Design review of the part built by this model. Coordinates are the model's own, in mm. Give positions to 0.01 mm unless a question says otherwise; leave off trailing zeros. Loops run counter-clockwise (first coordinate to the right, second up) from the corner with the lowest first, then second, coordinate; pieces in that order, holes last. Notation, with made-up numbers: M 55,51 L 111,51 A24 cw 111,63 Z; hole C -17.75,3.5 d7. An arc over 180 degrees is marked long. Answer as CSV lines item,"result".
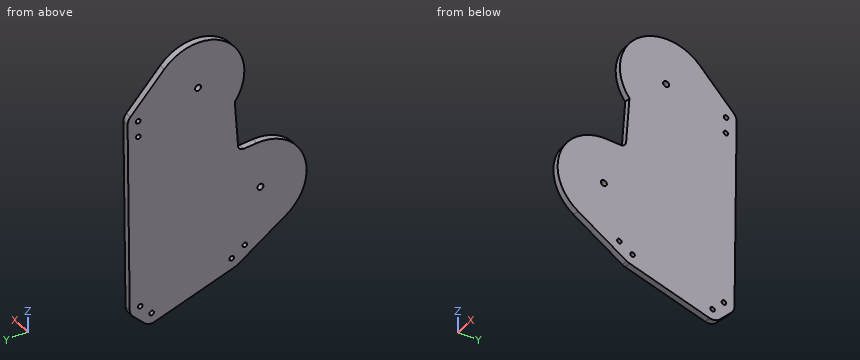
```python
from build123d import *

# Parameters (mm, degrees)
SKETCH1_R           = 1.7272
SKETCH1_R_2         = 2.25425
BOSS_EXTRUDE1_DEPTH = 4.953


with BuildPart() as part:
    # Sketch1 → Boss-Extrude1 (new body)
    with BuildSketch(Plane(origin=(0, 0, 0), x_dir=(0, 0, -1), z_dir=(1, 0, 0))):
        with BuildLine():
            Line((-353.601711985, 25.477997798), (-361.991932565, 34.057286733))
            ThreePointArc((-361.991932565, 34.057286733), (-364.547713568, 35.80650286), (-367.578343358, 36.444512791))
            Line((-367.578343358, 36.444512791), (-510.682190934, 38.038925927))
            ThreePointArc((-510.682190934, 38.038925927), (-513.636251412, 37.504085531), (-516.180391889, 35.910386439))
            Line((-516.180391889, 35.910386439), (-543.504008498, 10.46228671))
            ThreePointArc((-543.504008498, 10.46228671), (-546.343088738, -37.498931011), (-498.569252083, -42.597883175))
            Line((-498.569252083, -42.597883175), (-463.788130796, -45.097087093))
            ThreePointArc((-463.788130796, -45.097087093), (-461.050944436, -46.468361622), (-460.085098917, -49.373482176))
            Line((-460.085098917, -49.373482176), (-460.801802922, -59.347765878))
            ThreePointArc((-460.801802922, -59.347765878), (-437.483960059, -94.727435258), (-397.273694981, -81.364150349))
            Line((-397.273694981, -81.364150349), (-372.43498101, -44.703357168))
            ThreePointArc((-372.43498101, -44.703357168), (-371.88030639, -43.747530325), (-371.463761272, -42.723929302))
            Line((-371.463761272, -42.723929302), (-351.734061333, 17.455422825))
            ThreePointArc((-351.734061333, 17.455422825), (-351.545777131, 21.727936738), (-353.601711985, 25.477997798))
        make_face()
        with Locations((-359.276554144, 19.928216477)):
            Circle(SKETCH1_R, mode=Mode.SUBTRACT)
        with Locations((-367.666774725, 28.507505411)):
            Circle(SKETCH1_R, mode=Mode.SUBTRACT)
        with Locations((-510.7706223, 30.101918548)):
            Circle(SKETCH1_R, mode=Mode.SUBTRACT)
        with Locations((-379.006254083, -40.251135649)):
            Circle(SKETCH1_R, mode=Mode.SUBTRACT)
        with Locations((-426.087206182, -61.842189663)):
            Circle(SKETCH1_R_2, mode=Mode.SUBTRACT)
        with Locations((-519.783421193, -15.006500358)):
            Circle(SKETCH1_R_2, mode=Mode.SUBTRACT)
        with Locations((-385.737171654, -50.185658721)):
            Circle(SKETCH1_R, mode=Mode.SUBTRACT)
        with Locations((-498.771367049, 29.968227033)):
            Circle(SKETCH1_R, mode=Mode.SUBTRACT)
    extrude(amount=-BOSS_EXTRUDE1_DEPTH)


solid = part.part
```
1. We need section B-B, the plane y = -78. Write out the cut boundary in (x, z).
Answer block:
outline,"M -4.95,394.99 L 0,394.99 L 0,456.91 L -4.95,456.91 Z"
2. For P1, Ø1, axis at x = -1.5, y = -27.5, coming from the +Z side; P2, Ø1.5, axis at x = -2.5, z = 440, coming from the -Y side; P3, Ø1.5, axis at x = -1.5, y = -41.5, coming from the +Z side, all flat-tipped, find the tip position at first contact; note any pin that passes through.
Answer block:
P1,"z = 552.46"
P2,"y = -94.06"
P3,"z = 543.21"
3. We need section A-A, the plane x = -2.4. Count the separate pieces of the cut face and the enclosed holes in it, plus the area to 3 significant figures.
Answer block:
separate pieces,"1"
enclosed holes,"8"
area,"18,400 mm²"
4. To check wall thickness, follow L1, parallel to Z at x = -2, y = 30; L2, parallel to Z at x = -0.85, y = -60; L3, parallel to Z at x = -3.75, y = -39. State the ranges of each line that lie inside material, in increasing order. Write a range as [from, to].
Answer block:
L1,"[358.02, 366.8], [368.54, 497.04], [500.5, 509.05], [512.49, 522.53]"
L2,"[382.8, 424.79], [427.39, 460.84]"
L3,"[370.24, 377.82], [380.2, 545]"
5. We need section C-C, the plane z = 491. Write out the cut boundary in (x, y).
Answer block:
outline,"M -4.95,-43.14 L 0,-43.14 L 0,37.82 L -4.95,37.82 Z"
